```python
from build123d import *


with BuildPart() as part:
    # Sketch1 → Revolve1 (revolve)
    with BuildSketch(Plane(origin=(0, 0, 0), x_dir=(0, 0, -1), z_dir=(1, 0, 0)), mode=Mode.PRIVATE) as revolve1_sk:
        with BuildLine():
            Line((60.7822, -26.811732), (81.4578, -26.811732))
            Line((81.4578, -26.811732), (82.4611, -26.811732))
            Line((82.4611, -26.811732), (82.4611, -34.749232))
            Line((82.4611, -34.749232), (81.4578, -34.749232))
            Line((81.4578, -34.749232), (81.4578, -28.551632))
            Line((81.4578, -28.551632), (78.639993039, -28.551632))
            ThreePointArc((78.639993039, -28.551632), (77.1926569, -29.920339878), (75.5015, -30.973018125))
            Line((75.5015, -30.973018125), (75.5015, -33.555432))
            Line((75.5015, -33.555432), (66.7385, -33.555432))
            Line((66.7385, -33.555432), (66.7385, -30.973018125))
            ThreePointArc((66.7385, -30.973018125), (65.0473431, -29.920339878), (63.600006961, -28.551632))
            Line((63.600006961, -28.551632), (60.7822, -28.551632))
            Line((60.7822, -28.551632), (60.7822, -34.749232))
            Line((60.7822, -34.749232), (59.7789, -34.749232))
            Line((59.7789, -34.749232), (59.7789, -26.811732))
            Line((59.7789, -26.811732), (60.7822, -26.811732))
        make_face()
    revolve(revolve1_sk.sketch.rotate(Axis((0, -22.049232, -82.136173087), (0, 0, -1)), 270), axis=Axis((0, -22.049232, -82.136173087), (0, 0, -1)))


solid = part.part
```
Work out the finished part from the listing and answer in its coordinate system (mm). A direction names the side the tool comes from. Coordinates: 2 decimals unless noted, no trailing zeros. Loops run counter-clockwise (first coordinate to the right, second up) from the corner with the lowest first, then second, coordinate; pieces in that order, holes last. Notation, with made-up numbers: (-2, 5) - (53, 5) arc R18 ccw to (53, 13) - close; hole circle Ø1 at (-6.5, -2.75). An arc over 180 degrees is marked (long way). Use a Markdown table: item, result.
Item 1: Find section B-B, the plane y = -12. Determine the outline of the cut face in (x, z).
Evaluation:
| item | result |
|---|---|
| outline | (-7.77, -82.46) - (7.77, -82.46) - (7.77, -81.46) - (-7.77, -81.46) - close; (-7.77, -60.78) - (7.77, -60.78) - (7.77, -59.78) - (-7.77, -59.78) - close; (-5.6, -75.5) - (5.6, -75.5) - (5.6, -66.74) - (-5.6, -66.74) - close |
Item 2: The mould has two halves that part along Z. Classify faces 3 (the flat face through (-6, -15, -75.502)), 4 (the cylindrical face through (-1.65, -34.64, -81.95)), 5 (the flat face through (0, -17, -82.461)): +Z half, -Z half, draft (parallel to the pull), parting line (faces both ways), or undercut.
Evaluation:
| item | result |
|---|---|
| face 3 | undercut |
| face 4 | draft |
| face 5 | -Z half |
Item 3: For faces 1 (the flat face through (-6, -25, -81.458)), 2 (the cylindrical face through (-0.62, -26.77, -71.28)), determine the directions among +Z, -Z, +X, -X, +Y, -Y from which every point of the face is accessible in a straight line to the end or side of a thin tool.
Evaluation:
| item | result |
|---|---|
| face 1 | none |
| face 2 | +Z, -Z |
Item 4: Find section C-C, the plane x = -7.5. Determine the outline of the cut face in (y, z).
Evaluation:
| item | result |
|---|---|
| outline | (-32.3, -82.46) - (-11.8, -82.46) - (-11.8, -81.46) - (-32.3, -81.46) - close; (-32.3, -60.78) - (-11.8, -60.78) - (-11.8, -59.78) - (-32.3, -59.78) - close; (-30.78, -75.5) - (-26.88, -75.5) arc R6.53 ccw to (-17.21, -75.5) - (-13.32, -75.5) - (-13.32, -66.74) - (-17.21, -66.74) arc R6.53 ccw to (-26.88, -66.74) - (-30.78, -66.74) - close |
Item 5: Find section D-D, the plane z = -63.25. Determine the outline of the cut face in (x, y) (1 decimal).
Evaluation:
| item | result |
|---|---|
| outline | circle Ø13 at (0, -22); hole circle Ø9.5 at (0, -22) |
Item 6: Given pin 1 Ø6 at (y, z) = (-24.5, -69) entering from -X; pin 2 Ø6 at (y, z) = (-12.5, -69) entering from +X; pin 3 Ø5 at (y, z) = (-23.5, -63) entering from +X, each flat-ended and moving along its own axis, determine where each tip first touches the part or whether it passes through.
Evaluation:
| item | result |
|---|---|
| pin 1 | stops at x = -11.51 |
| pin 2 | stops at x = 9.46 |
| pin 3 | stops at x = 12.7 |
Item 7: Find section A-A, the plane x = 0. Determine the outline of the cut face in (y, z).
Evaluation:
| item | result |
|---|---|
| outline | (-34.75, -82.46) - (-26.81, -82.46) - (-26.81, -59.78) - (-34.75, -59.78) - (-34.75, -60.78) - (-28.55, -60.78) - (-28.55, -63.6) arc R9.94 ccw to (-30.97, -66.74) - (-33.56, -66.74) - (-33.56, -75.5) - (-30.97, -75.5) arc R9.94 ccw to (-28.55, -78.64) - (-28.55, -81.46) - (-34.75, -81.46) - close; (-17.29, -82.46) - (-9.35, -82.46) - (-9.35, -81.46) - (-15.55, -81.46) - (-15.55, -78.64) arc R9.94 ccw to (-13.13, -75.5) - (-10.54, -75.5) - (-10.54, -66.74) - (-13.13, -66.74) arc R9.94 ccw to (-15.55, -63.6) - (-15.55, -60.78) - (-9.35, -60.78) - (-9.35, -59.78) - (-17.29, -59.78) - close |
Item 8: Consider probe 1 along Z at (x, y) = (10.5, -19); probe 2 along Z at (x, y) = (4.5, -33); probe 3 along Y at (x, z) = (0, -69.5). Determine where each line is inside the solid, lowest interval first. Write a range as from..to.
Evaluation:
| item | result |
|---|---|
| probe 1 | z = -82.46..-81.46, -75.5..-66.74, -60.78..-59.78 |
| probe 2 | z = -82.46..-81.46, -60.78..-59.78 |
| probe 3 | y = -33.56..-26.81, -17.29..-10.54 |
